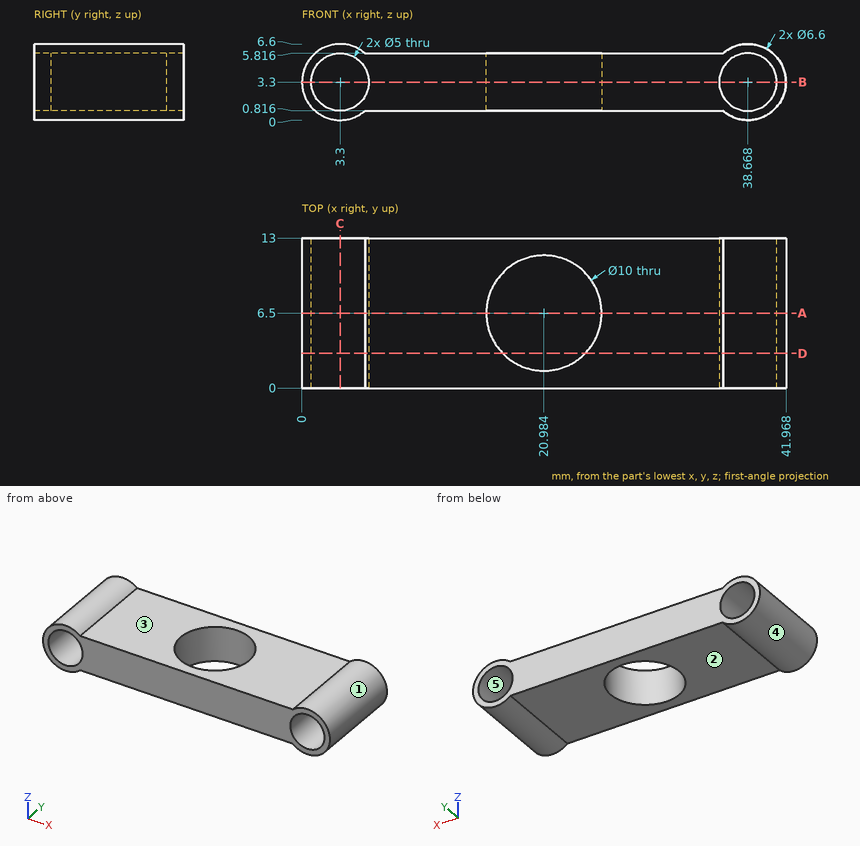
Drawing for the job (mm, zero at the part's lowest x, y, z). A direction names the side the tool comes from. Round coordinates to 2 decimals unless told otherwise and drop trailing zeros. Write each loop counter-clockwise with the first axis right and the second up, starting at its lowest first coordinate (ties: lowest second). Pieces come first, ordered by that corner, then holes. Notation, with made-up numbers: M 60.25,63 L 88.25,63 A23 cw 88.25,94 Z; hole C -5,8 d1. An arc over 180 degrees is marked long. Answer as a JSON object with one key per item and string values. Group by question number.
(1) Flat gauge pins, fed straight in: pin 1 (2 mm diameter, centred on x = 32, z = 5.5, fed in from -Y); pin 2 (3 mm diameter, centred on y = 10.5, z = 1, fed in from -X); pin 3 (4 mm diameter, centred on x = 17.5, y = 4, fed in from +Z); pin 4 (6.5 mm diameter, centred on x = 19.5, y = 9, fed in from -Z). Where does each tip first touch, or does it go through?
(2) Cut at C-C (x = 3.3). Give the cut face in (y, z), and give its area (3 significant figures).
(3) Cut at A-A (y = 6.5). Give the cut face in (x, z), and give its area (4 significant figures).
(4) Cut at D-D (y = 3). Give the cut face in (x, z), and give its area (3 significant figures).
(5) Cut at B-B (z = 3.3). Give the cut face in (x, y), and give its area (3 significant figures).
(6) Which spindle directions (+Z, -Z, +X, -X, +Y, -Y) get a long thin tool onto all of the face, cutting with end or side? Do the marked faces 1 and 2. Say none if no direction does.
(7) Mould opens along Z. For the marked faces 3, 4 and 5 say: pulls with the +Z half, pulls with the -Z half, needs draft (parallel to the pull), parting line crosses it, or undercut.
(8) Drill centre lines: L1, parallel to X at y = 10.5, z = 1.5 (1 decimal); L2, parallel to X at y = 6.75, z = 4.5 (1 decimal); L3, parallel to X at y = 12.25, z = 2.25. Where is each one in solid material? Low to high.
Responses:
{
 "1": {"pin 1": "stops at y = 0", "pin 2": "stops at x = 0.1", "pin 3": "stops at z = 5.82", "pin 4": "stops at z = 0.82"},
 "2": {"outline": "M 0,0 L 13,0 L 13,0.8 L 0,0.8 Z; M 0,5.8 L 13,5.8 L 13,6.6 L 0,6.6 Z", "area": "20.8 mm2"},
 "3": {"outline": "M 5.44,5.82 A3.3 ccw long 5.47,0.82 L 15.98,0.82 L 15.98,5.82 Z; M 25.98,0.82 L 36.5,0.82 A3.3 ccw long 36.53,5.82 L 25.98,5.82 Z; hole C 3.3,3.3 d5; hole C 38.67,3.3 d5", "area": "126.5 mm2"},
 "4": {"outline": "M 5.44,5.82 A3.3 ccw long 5.47,0.82 L 17.41,0.82 L 17.41,5.82 Z; M 24.55,0.82 L 36.5,0.82 A3.3 ccw long 36.53,5.82 L 24.55,5.82 Z; hole C 3.3,3.3 d5; hole C 38.67,3.3 d5", "area": "141 mm2"},
 "5": {"outline": "M 0,0 L 0.8,0 L 0.8,13 L 0,13 Z; M 5.8,0 L 36.17,0 L 36.17,13 L 5.8,13 Z; M 41.17,0 L 41.97,0 L 41.97,13 L 41.17,13 Z; hole C 20.98,6.5 d10", "area": "337 mm2"},
 "6": {"face 1": "+Y, -Y", "face 2": "-Z, +Y, -Y"},
 "7": {"face 3": "pulls with the +Z half", "face 4": "parting line crosses it", "face 5": "undercut"},
 "8": {"L1": "x = 0.5 to 1.6, 5 to 18, 24 to 36.9, 40.4 to 41.4", "L2": "x = 0.2 to 1.1, 5.5 to 16, 26 to 36.5, 40.9 to 41.7", "L3": "x = 0.17 to 1.03, 5.57 to 36.4, 40.94 to 41.8"}
}
